from build123d import *

# Parameters (mm, degrees)
DODANIE_WYCI_GNI_CIE1_DEPTH = 30
SKORUPA2_T                  = -4


with BuildPart() as part:
    # Szkic1 → Dodanie-wyciągnięcie1 (new body)
    with BuildSketch(Plane.XY):
        Polygon((-43.89930842, 241.108747994), (50.10069158, 241.108747994), (50.10069158, 18.932504013), (45.60069158, -76.067495987), (-39.39930842, -76.067495987), (-43.89930842, 18.932504013), align=None)
    extrude(amount=DODANIE_WYCI_GNI_CIE1_DEPTH)

    # Skorupa2
    skorupa2_openings = [part.faces().sort_by_distance(p)[0] for p in [
        (3.10069158, 241.108747994, 15),
        (3.10069158, -76.067495987, 15),
        (3.10069158, 84.366979784, 0),
    ]]
    offset(amount=SKORUPA2_T, openings=skorupa2_openings, kind=Kind.INTERSECTION)


solid = part.part
Could you check a few things on this model? Use its own coordinates, in mm. A direction names the side the tool comes from. Coordinates: 2 decimals unless noted, no trailing zeros. Order: outer loops, then holes, each group sorted by start corner. A loop starts at its lowest first (then second) coordinate and runs counter-clockwise, first axis right, second up. Notation, with made-up numbers: (-24, 16.25) - (23, 16.25) arc R25 ccw to (23, 42.25) - close; hole circle Ø8 at (19, -18). An arc over 180 degrees is marked (long way). Answer in a Markdown table with one row per item. Add a question column.
(1) If we section it at B-B, the plane y = 187: Please give me the cut outline in (x, z).
(2) If we section it at A-A, the plane z = 10: Please give me the cut outline in (x, y), then the cut area to 3 significant figures.
(3) Will these pins go through, and if not, where does the flat tip stop? pin 1 (12 mm diameter, centred on y = -10, z = 19.5, fed in from -X); pin 2 (2 mm diameter, centred on x = 32, y = 190, fed in from -Z).
(4) If we section it at D-D, the plane y = -5: Please give me the cut outline in (x, z).
(5) On a 3-axis mill with a long thin cutter (end or side, diameter ignored), from which of +Z, -Z, +X, -X, +Y, -Y can I reach the whole of each face in a straight line? I mean faces 1 (the face through (43.88, -27.85, 12.82)), 2 (the face through (-43.899, 128, 15)). Say none if no direction works.
(6) If we mould it in two halves opening along X, with no side actions, what happens to faces 3 (the face through (47.882, -27.902, 14.79)), 4 (the face through (-39.899, 129, 13)), 5 (the face through (3, -76.067, 27)), 6 (the face through (-41.618, -29.232, 14.79))? For each: released by +X, released by -X, zero draft, split by the parting line, or undercut.
(7) I need wall thicknesses on L1, parallel to X at y = 153.5, z = 20.5; L2, parallel to Z at x = -32, y = -59.5; L3, parallel to X at y = -55.5, z = 14.25. Which ranges of each line are inside material? Lowest first, please.
(8) If we section it at C-C, the plane x = -12: Please give me the cut outline in (y, z), then the cut area to 3 significant figures.
Results are:
| question | item | result |
|---|---|---|
| 1 | outline | (-43.9, 0) - (-39.9, 0) - (-39.9, 26) - (46.1, 26) - (46.1, 0) - (50.1, 0) - (50.1, 30) - (-43.9, 30) - close |
| 2 | outline | (-43.9, 18.93) - (-39.4, -76.07) - (-35.39, -76.07) - (-39.9, 19.03) - (-39.9, 241.11) - (-43.9, 241.11) - close; (41.6, -76.07) - (45.6, -76.07) - (50.1, 18.93) - (50.1, 241.11) - (46.1, 241.11) - (46.1, 19.03) - close |
| 2 | area | 2,540 mm2 |
| 3 | pin 1 | stops at x = -42.81 |
| 3 | pin 2 | stops at z = 26 |
| 4 | outline | (-42.77, 0) - (-38.76, 0) - (-38.76, 26) - (44.96, 26) - (44.96, 0) - (48.97, 0) - (48.97, 30) - (-42.77, 30) - close |
| 5 | face 1 | -Z, +Y |
| 5 | face 2 | +Z, -Z, -X, +Y, -Y |
| 6 | face 3 | released by +X |
| 6 | face 4 | undercut |
| 6 | face 5 | zero draft |
| 6 | face 6 | released by -X |
| 7 | L1 | x = -43.9 to -39.9, 46.1 to 50.1 |
| 7 | L2 | z = 26 to 30 |
| 7 | L3 | x = -40.37 to -36.37, 42.57 to 46.57 |
| 8 | outline | (-76.07, 26) - (241.11, 26) - (241.11, 30) - (-76.07, 30) - close |
| 8 | area | 1,270 mm2 |
